```python
from build123d import *

# Parameters (mm, degrees)
SKETCH1_R           = 0.9
SKETCH1_R_2         = 7.5
SKETCH1_R_3         = 1
BOSS_EXTRUDE1_DEPTH = 1.5
FILLET1_R           = 0.5


with BuildPart() as part:
    # Sketch1 → Boss-Extrude1 (new body)
    with BuildSketch(Plane(origin=(0, 0, 0), x_dir=(1, 0, 0), z_dir=(0, 1, 0))):
        with BuildLine():
            Line((-3, -12.1346611), (-3, -12.5))
            ThreePointArc((-3, -12.5), (0, -15.5), (3, -12.5))
            Line((3, -12.5), (3, -12.1346611))
            ThreePointArc((3, -12.1346611), (6.25, -10.825317547), (9.008924778, -8.665406761))
            Line((9.008924778, -8.665406761), (9.325317547, -8.848076211))
            ThreePointArc((9.325317547, -8.848076211), (13.423393759, -7.75), (12.325317547, -3.651923789))
            Line((12.325317547, -3.651923789), (12.008924778, -3.469254338))
            ThreePointArc((12.008924778, -3.469254338), (12.5, 0), (12.008924778, 3.469254338))
            Line((12.008924778, 3.469254338), (12.325317547, 3.651923789))
            ThreePointArc((12.325317547, 3.651923789), (13.423393759, 7.75), (9.325317547, 8.848076211))
            Line((9.325317547, 8.848076211), (9.008924778, 8.665406761))
            ThreePointArc((9.008924778, 8.665406761), (6.25, 10.825317547), (3, 12.1346611))
            Line((3, 12.1346611), (3, 12.5))
            ThreePointArc((3, 12.5), (0, 15.5), (-3, 12.5))
            Line((-3, 12.5), (-3, 12.1346611))
            ThreePointArc((-3, 12.1346611), (-6.25, 10.825317547), (-9.008924778, 8.665406761))
            Line((-9.008924778, 8.665406761), (-9.325317547, 8.848076211))
            ThreePointArc((-9.325317547, 8.848076211), (-13.423393759, 7.75), (-12.325317547, 3.651923789))
            Line((-12.325317547, 3.651923789), (-12.008924778, 3.469254338))
            ThreePointArc((-12.008924778, 3.469254338), (-12.5, 0), (-12.008924778, -3.469254338))
            Line((-12.008924778, -3.469254338), (-12.325317547, -3.651923789))
            ThreePointArc((-12.325317547, -3.651923789), (-13.423393759, -7.75), (-9.325317547, -8.848076211))
            Line((-9.325317547, -8.848076211), (-9.008924778, -8.665406761))
            ThreePointArc((-9.008924778, -8.665406761), (-6.25, -10.825317547), (-3, -12.1346611))
        make_face()
        with Locations(Location((-10.825317547, -6.25, 0), (0, 0, 270))):
            Circle(SKETCH1_R, mode=Mode.SUBTRACT)
        with Locations(Location((0, 0, 0), (0, 0, 270))):
            Circle(SKETCH1_R_2, mode=Mode.SUBTRACT)
        with Locations(Location((-10.825317547, 6.25, 0), (0, 0, 270))):
            Circle(SKETCH1_R_3, mode=Mode.SUBTRACT)
        with Locations(Location((0, 12.5, 0), (0, 0, 270))):
            Circle(SKETCH1_R, mode=Mode.SUBTRACT)
        with Locations(Location((10.825317547, 6.25, 0), (0, 0, 270))):
            Circle(SKETCH1_R_3, mode=Mode.SUBTRACT)
        with Locations(Location((10.825317547, -6.25, 0), (0, 0, 270))):
            Circle(SKETCH1_R, mode=Mode.SUBTRACT)
        with Locations(Location((0, -12.5, 0), (0, 0, 270))):
            Circle(SKETCH1_R_3, mode=Mode.SUBTRACT)
    extrude(amount=BOSS_EXTRUDE1_DEPTH)

    # Fillet1
    fillet1_edges = [part.edges().sort_by_distance(p)[0] for p in [
        (-3, 0.75, 12.1346611),
        (3, 0.75, 12.1346611),
        (9.008924778, 0.75, 8.665406761),
        (12.008924778, 0.75, 3.469254338),
        (12.008924778, 0.75, -3.469254338),
        (9.008924778, 0.75, -8.665406761),
        (3, 0.75, -12.1346611),
        (-3, 0.75, -12.1346611),
        (-9.008924778, 0.75, -8.665406761),
        (-12.008924778, 0.75, -3.469254338),
        (-12.008924778, 0.75, 3.469254338),
        (-9.008924778, 0.75, 8.665406761),
    ]]
    fillet(fillet1_edges, radius=FILLET1_R)


solid = part.part
```
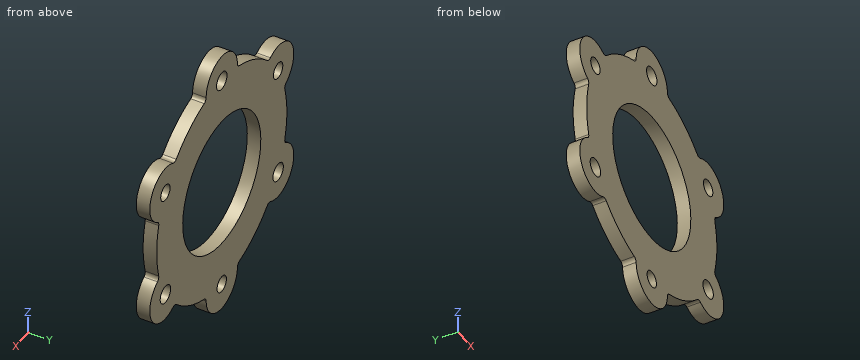
Read the model definition and answer for the solid it produces. Units are mm, in the model's axes. Coordinates: 2 decimals unless noted, no trailing zeros. Loops run counter-clockwise (first coordinate to the right, second up) from the corner with the lowest first, then second, coordinate; pieces in that order, holes last. Notation, with made-up numbers: (-15.5, 11) - (-7.5, 11) arc R24 cw to (-7.5, 24) - close; hole circle Ø2 at (-19.5, 69). An arc over 180 degrees is marked (long way). Answer in a Markdown table with one row per item.
1. Find section D-D, the plane x = 6. Write down the section's boundary in (y, z), then the cut area to 3 significant figures.
Conclusion:
| item | result |
|---|---|
| outline | (0, -10.97) - (1.5, -10.97) - (1.5, -4.5) - (0, -4.5) - close; (0, 4.5) - (1.5, 4.5) - (1.5, 10.97) - (0, 10.97) - close |
| area | 19.4 mm² |
2. Find section A-A, the plane x = 0. Write down the section's boundary in (y, z).
Conclusion:
| item | result |
|---|---|
| outline | (0, -15.5) - (1.5, -15.5) - (1.5, -13.4) - (0, -13.4) - close; (0, -11.6) - (1.5, -11.6) - (1.5, -7.5) - (0, -7.5) - close; (0, 7.5) - (1.5, 7.5) - (1.5, 11.5) - (0, 11.5) - close; (0, 13.5) - (1.5, 13.5) - (1.5, 15.5) - (0, 15.5) - close |
3. Given pin 1 (2.5 mm diameter, centred on x = 0, z = 12.5, fed in from +Y); pin 2 (1.1 mm diameter, centred on x = 0, z = -12.5, fed in from -Y), each flat-ended and moving along its own axis, determine where each tip first touches the part or whether it passes through.
Conclusion:
| item | result |
|---|---|
| pin 1 | stops at y = 1.5 |
| pin 2 | passes through |
4. Find section C-C, the plane z = -6.25. Write down the section's boundary in (x, y), then the cut area to 3 significant figures.
Conclusion:
| item | result |
|---|---|
| outline | (-13.83, 0) - (-11.83, 0) - (-11.83, 1.5) - (-13.83, 1.5) - close; (-9.83, 0) - (-4.15, 0) - (-4.15, 1.5) - (-9.83, 1.5) - close; (4.15, 0) - (9.83, 0) - (9.83, 1.5) - (4.15, 1.5) - close; (11.83, 0) - (13.83, 0) - (13.83, 1.5) - (11.83, 1.5) - close |
| area | 23.0 mm² |
5. Straight lines are drawn through the part: line 1 (X direction, y = 0.6, z = -12.5); line 2 (X direction, y = 1.2, z = -6.25); line 3 (Z direction, x = 11.25, y = 0.7). For each, find the intervals that lie inside material, in ascending order.
Conclusion:
| item | result |
|---|---|
| line 1 | x = -3 to -0.9, 0.9 to 3 |
| line 2 | x = -13.83 to -11.83, -9.83 to -4.15, 4.15 to 9.83, 11.83 to 13.83 |
| line 3 | z = -9.22 to -7.16, -5.34 to 5.46, 7.04 to 9.22 |
6. Find section B-B, the plane z = 0. Write down the section's boundary in (x, y).
Conclusion:
| item | result |
|---|---|
| outline | (-12.5, 0) - (-7.5, 0) - (-7.5, 1.5) - (-12.5, 1.5) - close; (7.5, 0) - (12.5, 0) - (12.5, 1.5) - (7.5, 1.5) - close |
